from build123d import *


with BuildPart() as part:
    # Esboço2 → Revolução1 (revolve)
    with BuildSketch(Plane.XY, mode=Mode.PRIVATE) as revolu_o1_sk:
        Polygon((10, 0), (2.5, 0), (2.5, 4), (10, 4), (10, 3), (9, 2), (10, 1), align=None)
    revolve(revolu_o1_sk.sketch.rotate(Axis((0, 15.525574547, 0), (0, -1, 0)), 180), axis=Axis((0, 15.525574547, 0), (0, -1, 0)))


solid = part.part
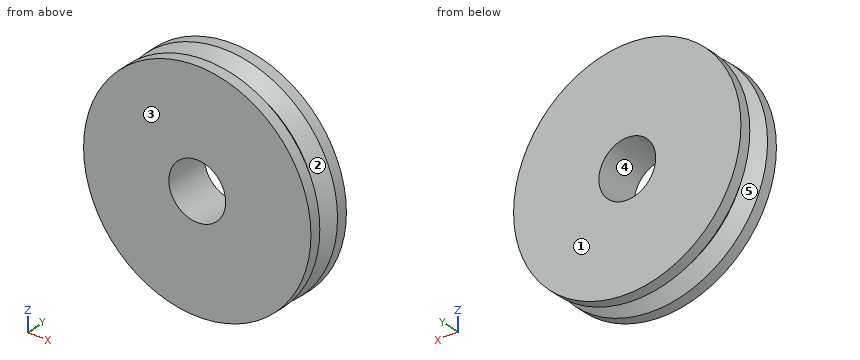
Work out the finished part from the listing and answer in its coordinate system (mm). Face numbers are marked on the shaded views. A direction names the side the tool comes from. Give positions to 0.01 mm unless a question says otherwise; leave off trailing zeros. Loops run counter-clockwise (first coordinate to the right, second up) from the corner with the lowest first, then second, coordinate; pieces in that order, holes last. Notation, with made-up numbers: (15, 70.5) -> (54, 70.5) arc R30 ccw to (54, 105.5) -> close; hole circle Ø4 at (4, 37.25). An arc over 180 degrees is marked (long way). Use a Markdown table: item, result. Add a question column.
1. Section A-A on z = 0 is taken. Determine the outline of the cut face in (x, y), and give its area (3 significant figures).
2. Find the intervals of material crossed by probe 1 along Z at (x, y) = (0, 1.85); probe 2 along Z at (x, y) = (0, 2.75); probe 3 along Z at (x, y) = (4, 3.45), in increasing order.
3. Section C-C on y = 1.5 is taken. Determine the outline of the cut face in (x, z), and give its area (3 significant figures).
4. Section D-D on y = 2.65 is taken. Determine the outline of the cut face in (x, z).
5. Section B-B on x = 0 is taken. Determine the outline of the cut face in (y, z).
6. Determine the mould class of the marked faces 1, 2 and 3 for opening direction Y: released by +Y, released by -Y, zero draft, split by the parting line, or undercut.
7. For the marked faces 4 and 5, determine the directions among +Z, -Z, +X, -X, +Y, -Y from which every point of the face is accessible in a straight line to the end or side of a thin tool.
Results below:
| question | item | result |
|---|---|---|
| 1 | outline | (-10, 0) -> (-2.5, 0) -> (-2.5, 4) -> (-10, 4) -> (-10, 3) -> (-9, 2) -> (-10, 1) -> close; (2.5, 0) -> (10, 0) -> (10, 1) -> (9, 2) -> (10, 3) -> (10, 4) -> (2.5, 4) -> close |
| 1 | area | 58.0 mm^2 |
| 2 | probe 1 | z = -9.15 to -2.5, 2.5 to 9.15 |
| 2 | probe 2 | z = -9.75 to -2.5, 2.5 to 9.75 |
| 2 | probe 3 | z = -9.17 to 9.17 |
| 3 | outline | circle Ø19 at (0, 0); hole circle Ø5 at (0, 0) |
| 3 | area | 264 mm^2 |
| 4 | outline | circle Ø19.3 at (0, 0); hole circle Ø5 at (0, 0) |
| 5 | outline | (0, -10) -> (1, -10) -> (2, -9) -> (3, -10) -> (4, -10) -> (4, -2.5) -> (0, -2.5) -> close; (0, 2.5) -> (4, 2.5) -> (4, 10) -> (3, 10) -> (2, 9) -> (1, 10) -> (0, 10) -> close |
| 6 | face 1 | released by +Y |
| 6 | face 2 | undercut |
| 6 | face 3 | released by -Y |
| 7 | face 4 | +Y, -Y |
| 7 | face 5 | none |
